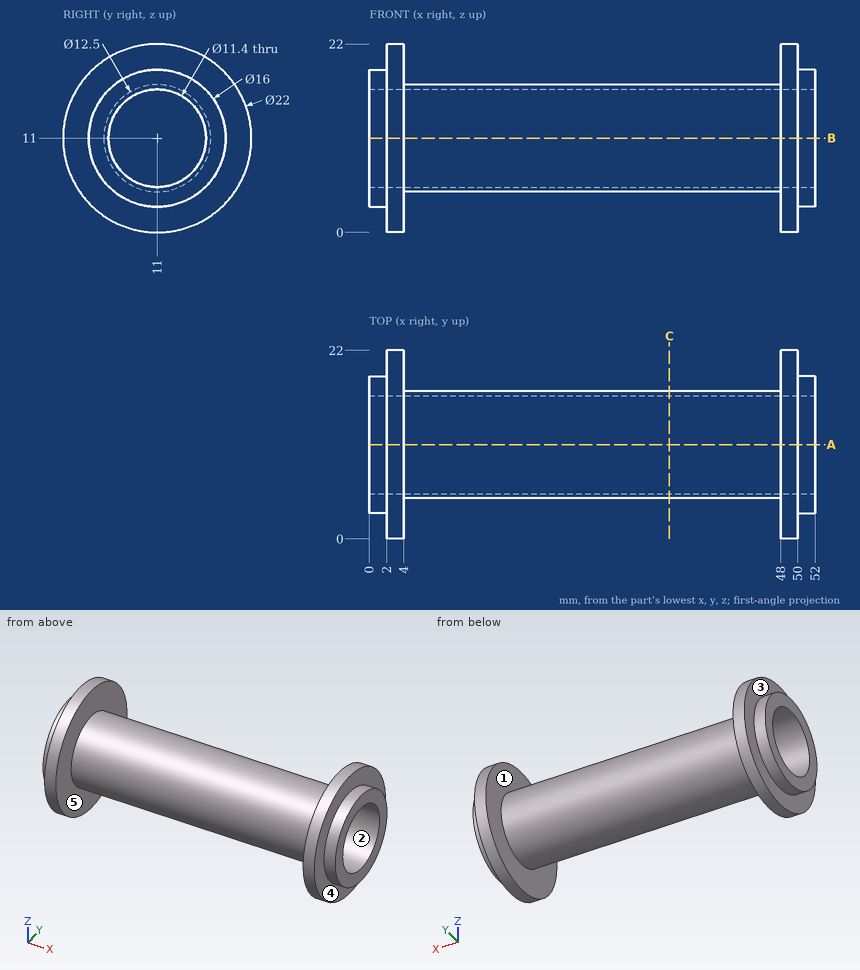
The drawing under review shows one solid part. Ordinate dimensions are in mm from its lowest x, y, z. A direction names the side the tool comes from. Round coordinates to 2 decimals unless told otherwise and drop trailing zeros. Loops run counter-clockwise (first coordinate to the right, second up) from the corner with the lowest first, then second, coordinate; pieces in that order, holes last.
Item 1: Clearance check with flat-ended pins moving along their axes: pin 1 Ø9 at (y, z) = (11, 11) entering from +X; pin 2 Ø6 at (x, y) = (11.5, 2.5) entering from +Z; pin 3 Ø5 at (x, z) = (33.5, 7) entering from +Y; pin 4 Ø6 at (x, z) = (23.5, 3.5) entering from +Y. State where each tip first meets the part, or that it passes through.
Determined:
pin 1: passes through
pin 2: stops at z = 13.97
pin 3: stops at y = 17.07
pin 4: stops at y = 15.34
Item 2: Take a section at C-C (x = 35). Write out the cut boundary in (y, z), then the cut area to 3 significant figures.
Determined:
outline: circle Ø12.5 at (11, 11); hole circle Ø11.4 at (11, 11)
area: 20.6 mm2
Item 3: For line 1 (Z direction, x = 15, y = 11); line 2 (X direction, y = 10.75, z = 2); line 3 (X direction, y = 3.5, z = 10.5), list the stretches that pass through material, from the lowest coordinate up.
Determined:
line 1: z = 4.75 to 5.3, 16.7 to 17.25
line 2: x = 2 to 4, 48 to 50
line 3: x = 0 to 4, 48 to 52
Item 4: Take a section at A-A (y = 11). Write out the cut boundary in (x, z), then the cut area to 3 significant figures.
Determined:
outline: (0, 3) - (2, 3) - (2, 0) - (4, 0) - (4, 4.75) - (48, 4.75) - (48, 0) - (50, 0) - (50, 3) - (52, 3) - (52, 5.3) - (0, 5.3) - close; (0, 16.7) - (52, 16.7) - (52, 19) - (50, 19) - (50, 22) - (48, 22) - (48, 17.25) - (4, 17.25) - (4, 22) - (2, 22) - (2, 19) - (0, 19) - close
area: 109 mm2
Item 5: Mouldability with a two-part tool opening along X and no side actions: class the marked faces 1, 2 and 3 as released by +X, released by -X, zero draft, split by the parting line, or undercut.
Determined:
face 1: undercut
face 2: zero draft
face 3: released by -X
Item 6: For the marked faces 4 and 5, list the 3-axis set-ups (+Z, -Z, +X, -X, +Y, -Y) from which the entire face can be reached by the end or side of a thin tool; tool diameter is ignored.
Determined:
face 4: +X
face 5: none
